For this review, take the finished solid that the model builds, in its own axes (mm). A direction names the side the tool comes from. Round coordinates to 2 decimals unless told otherwise and drop trailing zeros. Write each loop counter-clockwise with the first axis right and the second up, starting at its lowest first coordinate (ties: lowest second). Pieces come first, ordered by that corner, then holes. Notation, with made-up numbers: (57, 2.5) -> (104, 2.5) arc R26 ccw to (104, 33.5) -> close; hole circle Ø8 at (37, 56.25). An arc over 180 degrees is marked (long way). Answer in a Markdown table with one row per item. Add a question column.
```python
from build123d import *

# Parameters (mm, degrees)
BASE_FLANGE1_DEPTH = 16
SKETCH6_R          = 1.984375
SKETCH6_R_2        = 3.175
CUT_EXTRUDE1_DEPTH = 117.622837005


# Sheet-metal steps are written as plain solids
with BuildPart() as part:
    # Sketch1 → Base-Flange1 (new, symmetric)
    with BuildSketch(Plane.XY):
        with BuildLine():
            Line((-60, 0), (-40.601431382, 0))
            ThreePointArc((-40.601431382, 0), (-40.135564637, 0.166032093), (-39.879713724, 0.58928))
            Line((-39.879713724, 0.58928), (-20.240572553, 96.801029711))
            ThreePointArc((-20.240572553, 96.801029711), (-19.728870727, 97.647525524), (-18.797137237, 97.979589711))
            Line((-18.797137237, 97.979589711), (18.797137237, 97.979589711))
            ThreePointArc((18.797137237, 97.979589711), (19.728870727, 97.647525524), (20.240572553, 96.801029711))
            Line((20.240572553, 96.801029711), (39.879713724, 0.58928))
            ThreePointArc((39.879713724, 0.58928), (40.135564637, 0.166032093), (40.601431382, 0))
            Line((40.601431382, 0), (60, 0))
            Line((60, 0), (60, -0.7366))
            Line((60, -0.7366), (40.601431382, -0.7366))
            ThreePointArc((40.601431382, -0.7366), (39.669697892, -0.404535813), (39.157996066, 0.44196))
            Line((39.157996066, 0.44196), (19.518854895, 96.653709711))
            ThreePointArc((19.518854895, 96.653709711), (19.263003982, 97.076957618), (18.797137237, 97.242989711))
            Line((18.797137237, 97.242989711), (-18.797137237, 97.242989711))
            ThreePointArc((-18.797137237, 97.242989711), (-19.263003982, 97.076957618), (-19.518854895, 96.653709711))
            Line((-19.518854895, 96.653709711), (-39.157996066, 0.44196))
            ThreePointArc((-39.157996066, 0.44196), (-39.669697892, -0.404535813), (-40.601431382, -0.7366))
            Line((-40.601431382, -0.7366), (-60, -0.7366))
            Line((-60, -0.7366), (-60, 0))
        make_face()
    extrude(amount=BASE_FLANGE1_DEPTH, both=True)

    # Sketch6 → Cut-Extrude1 (cut, through all)
    with BuildSketch(Plane(origin=(0, 97.979589711, 0), x_dir=(1, 0, 0), z_dir=(0, 1, 0))):
        with Locations(Location((-50, 6, 0), (0, 0, 270))):
            Circle(SKETCH6_R)
        with Locations(Location((-50, -6, 0), (0, 0, 270))):
            Circle(SKETCH6_R)
        with Locations(Location((0, 0, 0), (0, 0, 270))):
            Circle(SKETCH6_R_2)
        with Locations(Location((50, -6, 0), (0, 0, 180))):
            Circle(SKETCH6_R)
        with Locations(Location((50, 6, 0), (0, 0, 180))):
            Circle(SKETCH6_R)
    extrude(amount=-CUT_EXTRUDE1_DEPTH, mode=Mode.SUBTRACT)


solid = part.part
```
1. The part is to be moulded in two halves that separate along Z. For faces 1 (the flat face through (-29.2, 49.22, 0.22)), 2 (the cylindrical face through (-48.033, -0.363, 5.742)), say which applies: pulls with the +Z half, pulls with the -Z half, needs draft (parallel to the pull), parting line crosses it, or undercut.
2. For L1, parallel to Y at x = -54.5, z = 7.5; L2, parallel to Y at x = -3, z = 2; L3, parallel to X at y = 11, z = 13, list the stretches that pass through material, from the lowest coordinate up. Write a range as [from, to].
3. We need section D-D (x = 50). Write out the cut boundary in (y, z).
4. We need section A-A (x = 0). Write out the cut boundary in (y, z) (3 decimals).
5. We need section B-B (z = 0). Write out the cut boundary in (x, y) (3 decimals).
6. We need section C-C (y = 33). Write out the cut boundary in (x, z), plus the area to 3 significant figures.
7. Clearance check with flat-ended pins moving along their axes: pin 1 Ø8 at (x, z) = (-7.5, -4.5) entering from -Y; pin 2 Ø3 at (x, z) = (-50, 6) entering from -Y; pin 3 Ø4.5 at (x, z) = (50, 6) entering from -Y; pin 4 Ø12 at (y, z) = (31, 11) entering from -X. State where each tip first meets the part, or that it passes through.
8. Tool access review of faces 3 (the flat face through (-50, 0, 0)), 4 (the flat face through (50, 0, 0)), 5 (the flat face through (29.476, 47.874, 0.224)): name each direction out of +Z, -Z, +X, -X, +Y, -Y from which nothing blocks a thin tool from reaching the whole face with its end or side.
Response:
| question | item | result |
|---|---|---|
| 1 | face 1 | needs draft |
| 1 | face 2 | undercut |
| 2 | L1 | [-0.74, 0] |
| 2 | L2 | [97.24, 97.98] |
| 2 | L3 | [-37.75, -37], [37, 37.75] |
| 3 | outline | (-0.74, -16) -> (0, -16) -> (0, -7.98) -> (-0.74, -7.98) -> close; (-0.74, -4.02) -> (0, -4.02) -> (0, 4.02) -> (-0.74, 4.02) -> close; (-0.74, 7.98) -> (0, 7.98) -> (0, 16) -> (-0.74, 16) -> close |
| 4 | outline | (97.243, -16) -> (97.98, -16) -> (97.98, -3.175) -> (97.243, -3.175) -> close; (97.243, 3.175) -> (97.98, 3.175) -> (97.98, 16) -> (97.243, 16) -> close |
| 5 | outline | (-60, -0.737) -> (-40.601, -0.737) arc R1.473 ccw to (-39.158, 0.442) -> (-19.519, 96.654) arc R0.737 cw to (-18.797, 97.243) -> (-3.175, 97.243) -> (-3.175, 97.98) -> (-18.797, 97.98) arc R1.473 ccw to (-20.241, 96.801) -> (-39.88, 0.589) arc R0.737 cw to (-40.601, 0) -> (-60, 0) -> close; (3.175, 97.243) -> (18.797, 97.243) arc R0.737 cw to (19.519, 96.654) -> (39.158, 0.442) arc R1.473 ccw to (40.601, -0.737) -> (60, -0.737) -> (60, 0) -> (40.601, 0) arc R0.737 cw to (39.88, 0.589) -> (20.241, 96.801) arc R1.473 ccw to (18.797, 97.98) -> (3.175, 97.98) -> close |
| 6 | outline | (-33.26, -16) -> (-32.51, -16) -> (-32.51, 16) -> (-33.26, 16) -> close; (32.51, -16) -> (33.26, -16) -> (33.26, 16) -> (32.51, 16) -> close |
| 6 | area | 48.1 mm2 |
| 7 | pin 1 | y = 97.24 |
| 7 | pin 2 | through |
| 7 | pin 3 | y = -0.74 |
| 7 | pin 4 | x = -34.9 |
| 8 | face 3 | +Z, -Z, -X, +Y |
| 8 | face 4 | +Z, -Z, +X, +Y |
| 8 | face 5 | +Z, -Z, -Y |
